For this review, take the finished solid that the model builds, in its own axes (mm). Face numbers are marked on the shaded views. A direction names the side the tool comes from. Round coordinates to 2 decimals unless told otherwise and drop trailing zeros. Write each loop counter-clockwise with the first axis right and the second up, starting at its lowest first coordinate (ties: lowest second). Pieces come first, ordered by that corner, then holes. Notation, with made-up numbers: M 63.25,1 L 92.25,1 A23 cw 92.25,38 Z; hole C 51,4 d7. An arc over 180 degrees is marked long. One line per question, with ' | ' between items.
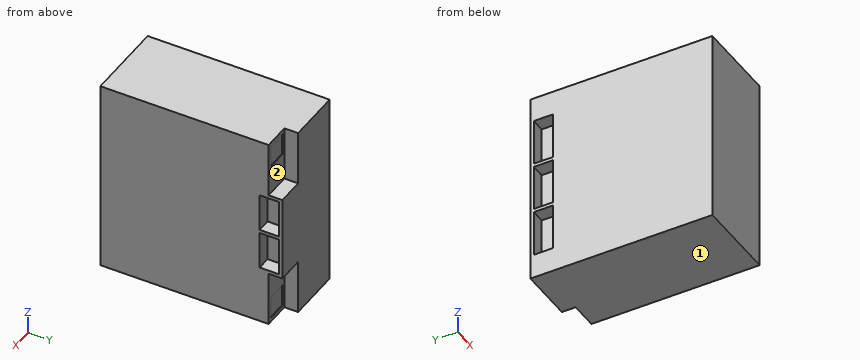
Autodesk Inventor part; units mm, degrees
ref_plane "YZ Plane" through (0, 0, 0) normal (1, 0, 0) x (0, 1, 0)
ref_plane "XZ Plane" through (0, 0, 0) normal (0, 1, 0) x (-1, 0, 0)
ref_plane "XY Plane" through (0, 0, 0) normal (0, 0, 1) x (1, 0, 0)
sketch "Sketch1" plane through (0, 0, 0) normal (0, 1, 0) x (-1, 0, 0)
  line L0 (0, 0) -> (76.2, 0)
  line L1 (76.2, 0) -> (76.2, -180.975)
  line L2 (76.2, -180.975) -> (0, -180.975)
  line L3 (0, -180.975) -> (0, 0)
  dimension "d0" = 76.2
  dimension "d1" = 180.975
extrude "Extrusion1" add sketch "Sketch1" along normal blind 168.275
sketch "Sketch2" plane through (0, 168.275, 0) normal (0, 1, 0) x (1, 0, 0)
  line L0 (-76.2, 0) -> (0, 0) construction
  line L1 (0, 0) -> (0, 180.975) construction
  line L2 (0, 180.975) -> (-76.2, 180.975) construction
  line L3 (-76.2, 180.975) -> (-76.2, 0) construction
  line L4 (0, 0) -> (0, 180.975)
  line L5 (0, 0) -> (-25.4, 0)
  line L6 (-25.4, 0) -> (-25.4, 50.8)
  line L7 (-25.4, 50.8) -> (0, 50.8)
  line L8 (0, 50.8) -> (0, 0)
  line L9 (0, 180.975) -> (-25.4, 180.975)
  line L10 (-25.4, 180.975) -> (-25.4, 130.175)
  line L11 (-25.4, 130.175) -> (0, 130.175)
  line L12 (0, 130.175) -> (0, 180.975)
  dimension "d4" = 25.4
  dimension "d5" = 50.8
  dimension "d6" = 25.4
  dimension "d7" = 50.8
extrude "Extrusion2" cut sketch "Sketch2" against normal blind 12.7
sketch "Sketch3" plane through (0, 0, 0) normal (1, 0, 0) x (0, 0, -1)
  line L0 (50.8, 168.275) -> (130.175, 168.275) construction
  line L1 (130.175, 155.575) -> (130.175, 168.275) construction
  line L2 (50.8, 168.275) -> (50.8, 155.575) construction
  line L3 (127, 155.575) -> (127, 165.1) construction
  line L4 (127, 165.1) -> (53.975, 165.1) construction
  line L5 (53.975, 165.1) -> (53.975, 155.575) construction
  line L6 (53.975, 165.1) -> (88.9, 165.1)
  line L7 (88.9, 165.1) -> (88.9, 147.32)
  line L8 (88.9, 147.32) -> (53.975, 147.32)
  line L9 (53.975, 147.32) -> (53.975, 165.1)
  line L10 (127, 165.1) -> (92.075, 165.1)
  line L11 (92.075, 165.1) -> (92.075, 147.32)
  line L12 (92.075, 147.32) -> (127, 147.32)
  line L13 (127, 147.32) -> (127, 165.1)
  point P0 (0, 0)
  dimension "d10" = 3.175
  dimension "d11" = 34.925
  dimension "d12" = 17.78
  dimension "d13" = 34.925
  dimension "d14" = 17.78
  dimension "d15" = 3.175
extrude "Extrusion3" cut sketch "Sketch3" against normal blind 12.7
sketch "Sketch4" plane through (0, 155.575, 0) normal (0, 1, 0) x (1, 0, 0)
  line L0 (0, 0) -> (-25.4, 0) construction
  line L1 (0, 50.8) -> (0, 0) construction
  line L2 (0, 180.975) -> (0, 130.175) construction
  line L3 (-25.4, 180.975) -> (0, 180.975) construction
  line L4 (-3.81, 50.8) -> (-3.81, 3.81) construction
  line L5 (-3.81, 3.81) -> (-25.4, 3.81) construction
  line L6 (-3.81, 130.175) -> (-3.81, 177.165) construction
  line L7 (-3.81, 177.165) -> (-25.4, 177.165) construction
  line L8 (-3.81, 3.81) -> (-22.86, 3.81)
  line L9 (-22.86, 3.81) -> (-22.86, 24.13)
  line L10 (-22.86, 24.13) -> (-3.81, 24.13)
  line L11 (-3.81, 24.13) -> (-3.81, 3.81)
  line L12 (-3.81, 177.165) -> (-22.86, 177.165)
  line L13 (-22.86, 177.165) -> (-22.86, 156.845)
  line L14 (-22.86, 156.845) -> (-3.81, 156.845)
  line L15 (-3.81, 156.845) -> (-3.81, 177.165)
  dimension "d18" = 3.81
  dimension "d19" = 3.81
  dimension "d20" = 19.05
  dimension "d21" = 20.32
  dimension "d22" = 19.05
  dimension "d23" = 20.32
extrude "Extrusion4" cut sketch "Sketch4" against normal blind 0.635
sketch "Sketch5" plane through (-76.2, 0, -180.975) normal (-1, 0, 0) x (0, 0, 1)
  line L0 (0, 168.275) -> (180.975, 168.275) construction
  line L1 (2.549, 165.1) -> (183.524, 165.1) construction
  line L2 (0, 0) -> (0, 168.275) construction
  line L3 (180.975, 0) -> (180.975, 168.275) construction
  line L4 (22.86, 2.1972) -> (22.86, 168.275) construction
  line L5 (158.115, 168.275) -> (158.115, 0) construction
  line L6 (22.86, 165.1) -> (66.04, 165.1)
  line L7 (66.04, 165.1) -> (66.04, 147.32)
  line L8 (66.04, 147.32) -> (22.86, 147.32)
  line L9 (22.86, 147.32) -> (22.86, 165.1)
  line L10 (158.115, 165.1) -> (114.935, 165.1)
  line L11 (114.935, 165.1) -> (114.935, 147.32)
  line L12 (114.935, 147.32) -> (158.115, 147.32)
  line L13 (158.115, 147.32) -> (158.115, 165.1)
  line L14 (66.04, 165.1) -> (69.215, 165.1) construction
  line L15 (114.935, 165.1) -> (111.76, 165.1) construction
  line L16 (69.215, 165.1) -> (111.76, 165.1)
  line L17 (111.76, 165.1) -> (111.76, 147.32)
  line L18 (111.76, 147.32) -> (69.215, 147.32)
  line L19 (69.215, 147.32) -> (69.215, 165.1)
  dimension "d26" = 3.175
  dimension "d27" = 22.86
  dimension "d28" = 22.86
  dimension "d29" = 43.18
  dimension "d30" = 43.18
  dimension "d31" = 17.78
  dimension "d32" = 3.175
  dimension "d33" = 3.175
  dimension "d34" = 42.545
  dimension "d35" = 17.78
extrude "Extrusion5" cut sketch "Sketch5" against normal blind 12.7
properties part number "Battery-1111-2017"
Item 1: Take a section at C-C (x = -16.5). Write out the cut boundary in (y, z) (3 decimals).
Results:
outline: M 0,-180.975 L 155.575,-180.975 L 155.575,-177.165 L 154.94,-177.165 L 154.94,-156.845 L 155.575,-156.845 L 155.575,-130.175 L 168.275,-130.175 L 168.275,-50.8 L 155.575,-50.8 L 155.575,-24.13 L 154.94,-24.13 L 154.94,-3.81 L 155.575,-3.81 L 155.575,0 L 0,0 Z
Item 2: Take a section at A-A (x = -68). Write out the cut boundary in (y, z) (3 decimals).
Results:
outline: M 0,-180.975 L 168.275,-180.975 L 168.275,0 L 0,0 Z; hole M 147.32,-158.115 L 165.1,-158.115 L 165.1,-114.935 L 147.32,-114.935 Z; hole M 147.32,-111.76 L 165.1,-111.76 L 165.1,-69.215 L 147.32,-69.215 Z; hole M 147.32,-66.04 L 165.1,-66.04 L 165.1,-22.86 L 147.32,-22.86 Z
Item 3: Insertion check: pin 1 Ø20.5 at (x, z) = (-7.5, -34.5) entering from +Y (3 decimals); pin 2 Ø14 at (y, z) = (157.5, -70) entering from +X; pin 3 Ø4 at (x, y) = (-17, 163) entering from -Z (3 decimals). Each pin has a flat end and moves straight along its axis. Give the tip position at first contact, or say it passes through.
Results:
pin 1: y = 155.575 | pin 2: x = -12.7 | pin 3: z = -130.175
Item 4: Machinability: for the marked faces 1 and 2, which of the approach directions +Z, -Z, +X, -X, +Y, -Y give a long, thin tool a straight path to every point of the face, cutting with its end or side? Answer none if there is none.
Results:
face 1: -Z, +X, -X, +Y, -Y | face 2: +Z, +X, +Y
Item 5: Take a section at B-B (z = -135.5). Write out the cut boundary in (x, y) (3 decimals).
Results:
outline: M -76.2,0 L 0,0 L 0,155.575 L -25.4,155.575 L -25.4,168.275 L -76.2,168.275 L -76.2,165.1 L -63.5,165.1 L -63.5,147.32 L -76.2,147.32 Z
Item 6: To check wall thickness, follow line 1 along Y through (x, z) = (-68, -140) (3 decimals); line 2 along Y through (x, z) = (-6.5, -141.5) (3 decimals); line 3 along Y through (x, z) = (-14, -169). State the ranges of each line that lie inside material, in increasing order. Write a range as from..to.
Results:
line 1: 0..147.32, 165.1..168.275 | line 2: 0..155.575 | line 3: 0..154.94
